Could you check a few things on this model? Use its own coordinates, in mm. Face numbers are marked on the shaded views. A direction names the side the tool comes from. Coordinates: 2 decimals unless noted, no trailing zeros. Loops run counter-clockwise (first coordinate to the right, second up) from the corner with the lowest first, then second, coordinate; pieces in that order, holes last.
1) Imagine slicing it at B-B on y = 9. Please give me the cut outline in (x, z).
2) Imagine slicing it at A-A on x = -8. Please give me the cut outline in (y, z).
3) Will these pins go through, and if not, where does the flat tip stop? P1, Ø5, axis at x = -0.5, z = -3, coming from the +Y side; P2, Ø1, axis at y = 19.5, z = -3.5, coming from the +X side; P3, Ø4, axis at y = 18.5, z = 0, coming from the +X side.
4) For the marked faces 3 and 4, which set-ups out of +Z, -Z, +X, -X, +Y, -Y let a thin tool reach every point of the face, with its end or its side?
5) If I drill on line 1 along X through (y, z) = (24, -5); line 2 along Y through (x, z) = (-1.5, -6); line 3 along X through (y, z) = (5.5, -1), over which ranges is the centre line in solid material (lowest first)?
6) Imagine slicing it at D-D on x = 4.25. Please give me the cut outline in (y, z).
7) Thinking about a two-plate mould opening in Z: for the marked faces 1 and 2, which applies, released by +Z, released by -Z, zero draft, split by the parting line, or undercut?
8) Imagine slicing it at C-C on z = 0.75. Please give me the cut outline in (x, y).
```python
from build123d import *

# Parameters (mm, degrees)
SKETCH_1_W      = 20
SKETCH_1_H      = 5
EXTRUDE_2_DEPTH = 2
SKETCH_4_R      = 1.5
EXTRUDE_3_DEPTH = 30


with BuildPart() as part:
    # 草图1 → 凸台-拉伸2 (new body)
    with BuildSketch(Plane(origin=(0, 0, 0), x_dir=(1, 0, 0), z_dir=(0, 1, 0))):
        Rectangle(SKETCH_1_W, SKETCH_1_H)
    extrude_2 = extrude(amount=-EXTRUDE_2_DEPTH)

    # 草图4 → 凸台-拉伸3 (add)
    with BuildSketch(Plane(origin=(0, 0, 0), x_dir=(1, 0, 0), z_dir=(0, 1, 0))):
        with Locations(Location((-8, 0, 0), (0, 0, 270))):
            Circle(SKETCH_4_R)
        with Locations(Location((8, 0, 0), (0, 0, 90))):
            Circle(SKETCH_4_R)
    extrude_3 = extrude(amount=EXTRUDE_3_DEPTH)

    # 镜向1: 凸台-拉伸2, 凸台-拉伸3 across plane
    add(extrude_2.mirror(Plane(origin=(0, 0, -2.5), x_dir=(1, 0, 0), z_dir=(0, 0, -1))))
    add(extrude_3.mirror(Plane(origin=(0, 0, -2.5), x_dir=(1, 0, 0), z_dir=(0, 0, -1))))


solid = part.part
```
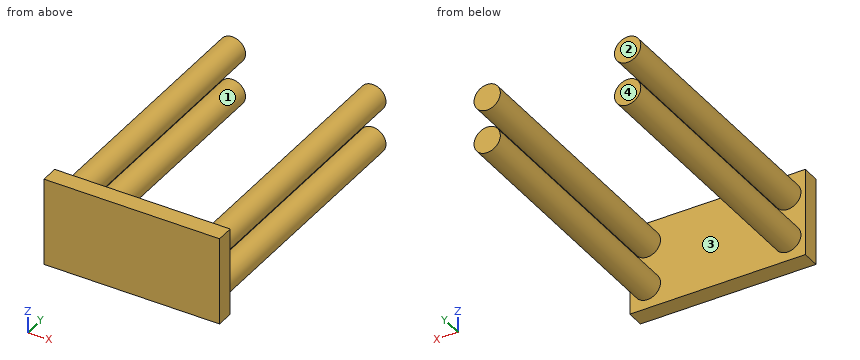
Filled in:
1. outline: circle Ø3 at (-8, -5); circle Ø3 at (-8, 0); circle Ø3 at (8, -5); circle Ø3 at (8, 0)
2. outline: (-2, -7.5) - (0, -7.5) - (0, -6.5) - (30, -6.5) - (30, -3.5) - (0, -3.5) - (0, -1.5) - (30, -1.5) - (30, 1.5) - (0, 1.5) - (0, 2.5) - (-2, 2.5) - close
3. P1: stops at y = 0
3. P2: stops at x = 9.12
3. P3: stops at x = 9.5
4. face 3: +Y
4. face 4: +Z, -Z, +X, -X, +Y
5. line 1: x = -9.5 to -6.5, 6.5 to 9.5
5. line 2: y = -2 to 0
5. line 3: x = -9.12 to -6.88, 6.88 to 9.12
6. outline: (-2, -7.5) - (0, -7.5) - (0, 2.5) - (-2, 2.5) - close
7. face 1: undercut
7. face 2: zero draft
8. outline: (-10, -2) - (10, -2) - (10, 0) - (9.3, 0) - (9.3, 30) - (6.7, 30) - (6.7, 0) - (-6.7, 0) - (-6.7, 30) - (-9.3, 30) - (-9.3, 0) - (-10, 0) - close
